from build123d import *

# Parameters (mm, degrees)
F0_W      = 50
F0_H      = 50
F2_W      = 50
F2_H      = 50
F4_R      = 5
F5_DEPTH  = 5
F6_R      = 5
F7_DEPTH  = 5
F9_R      = 5
F10_DEPTH = 5
F11_R     = 5
F12_DEPTH = 5


with BuildPart() as f3:
    # F0 (on Front) → F3 section 0
    with BuildSketch(Plane.XZ):
        with Locations((-25, 25)):
            Rectangle(F0_W, F0_H)
    # F2 (on offset) → F3 section 1
    with BuildSketch(Plane.XZ.offset(50)):
        with Locations((-25, 25)):
            Rectangle(F2_W, F2_H)
    loft()

    # F4 (on face) → F5 (cut)
    with BuildSketch(Plane.XZ.offset(50)):
        with Locations((-26.061153, 25.211331)):
            Circle(F4_R)
    extrude(amount=-F5_DEPTH, mode=Mode.SUBTRACT)

    # F6 (on face) → F7 (cut)
    with BuildSketch(Plane(origin=(0, 0, 0), x_dir=(1, 0, 0), z_dir=(0, 0, -1))):
        with Locations((-25, 25)):
            Circle(F6_R)
        with Locations((-37, 37)):
            Circle(F6_R)
        with Locations((-13, 37)):
            Circle(F6_R)
        with Locations((-13, 13)):
            Circle(F6_R)
        with Locations((-37, 13)):
            Circle(F6_R)
    extrude(amount=-F7_DEPTH, mode=Mode.SUBTRACT)

    # F9 (on face) → F10 (cut)
    with BuildSketch(Plane(origin=(0, 0, 0), x_dir=(-1, 0, 0), z_dir=(0, 1, 0))):
        with Locations((15.027642, 38.336441)):
            Circle(F9_R)
        with Locations((14.789439, 24.997041)):
            Circle(F9_R)
        with Locations((14.789439, 11.895845)):
            Circle(F9_R)
        with Locations((35.513151, 38.336441)):
            Circle(F9_R)
        with Locations((34.798544, 25.235245)):
            Circle(F9_R)
        with Locations((34.798544, 12.134047)):
            Circle(F9_R)
    extrude(amount=-F10_DEPTH, mode=Mode.SUBTRACT)

    # F11 (on face) → F12 (cut)
    with BuildSketch(Plane.XY.offset(50)):
        with Locations((-25, -37)):
            Circle(F11_R)
        with Locations((-25, -13)):
            Circle(F11_R)
    extrude(amount=-F12_DEPTH, mode=Mode.SUBTRACT)


solid = f3.part
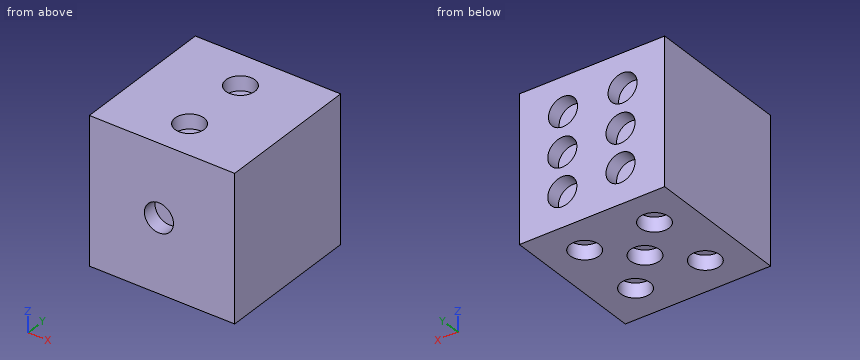
Here's how the part is built. I have some questions about the finished solid (model axes, mm). Coordinates: 2 decimals unless noted, no trailing zeros. Order: outer loops, then holes, each group sorted by start corner. A loop starts at its lowest first (then second) coordinate and runs counter-clockwise, first axis right, second up. Notation, with made-up numbers: M 16,-18 L 73,-18 A18 cw 73,14 Z; hole C 79,76 d6. An arc over 180 degrees is marked long. Answer as CSV lines item,"result". Start each with the question number.
1. I want a section at D-D, the plane z = 13. Write out the boundary of the cut face in (x, y), and give its area (3 significant figures).
2. For pin 1 (16 mm diameter, centred on x = -13, y = -13, fed in from -Z); pin 2 (8 mm diameter, centred on x = -25, y = -37, fed in from +Z); pin 3 (9 mm diameter, centred on x = -26.06, z = 25.21, fed in from -Y); pin 4 (5 mm diameter, centred on x = -15.5, z = 37.5, fed in from +Y), each with a flat end and sliding along its axis, tell me the tip position at first contact or that it passes through.
3. I want a section at A-A, the plane y = -13. Write out the boundary of the cut face in (x, z), and give its area (3 significant figures).
4. I need wall thicknesses on line 1 (X direction, y = -13, z = 1.9); line 2 (X direction, y = -1.5, z = 12). Which ranges of each line are inside material? Lowest first, please. Write a range as [from, to].
5. I want a section at C-C, the plane y = -25. Write out the boundary of the cut face in (x, z).
6. I want a section at B-B, the plane x = -35. Write out the boundary of the cut face in (y, z).
Recorded:
1,outline,"M -50,-50 L 0,-50 L 0,0 L -9.91,0 L -9.91,-5 L -19.67,-5 L -19.67,0 L -29.87,0 L -29.87,-5 L -39.72,-5 L -39.72,0 L -50,0 Z"
1,area,"2,400 mm2"
2,pin 1,"stops at z = 0"
2,pin 2,"stops at z = 45"
2,pin 3,"stops at y = -45"
2,pin 4,"stops at y = -5"
3,outline,"M -50,0 L -42,0 L -42,5 L -32,5 L -32,0 L -18,0 L -18,5 L -8,5 L -8,0 L 0,0 L 0,50 L -20,50 L -20,45 L -30,45 L -30,50 L -50,50 Z"
3,area,"2,350 mm2"
4,line 1,"x = [-50, -42], [-32, -18], [-8, 0]"
4,line 2,"x = [-50, -39.8], [-29.8, -19.79], [-9.79, 0]"
5,outline,"M -50,0 L -30,0 L -30,5 L -20,5 L -20,0 L 0,0 L 0,50 L -50,50 Z"
6,outline,"M -50,0 L -41.58,0 L -41.58,5 L -32.42,5 L -32.42,0 L -17.58,0 L -17.58,5 L -8.42,5 L -8.42,0 L 0,0 L 0,7.14 L -5,7.14 L -5,17.13 L 0,17.13 L 0,20.24 L -5,20.24 L -5,30.23 L 0,30.23 L 0,33.36 L -5,33.36 L -5,43.31 L 0,43.31 L 0,50 L -50,50 Z"
